Geometry check sheet. Reference: drawing and pictorial views, mm from the part's lowest x, y, z. A direction names the side the tool comes from. Give positions to 0.01 mm unless a question says otherwise; leave off trailing zeros. Order: outer loops, then holes, each group sorted by start corner. A loop starts at its lowest first (then second) coordinate and runs counter-clockwise, first axis right, second up.
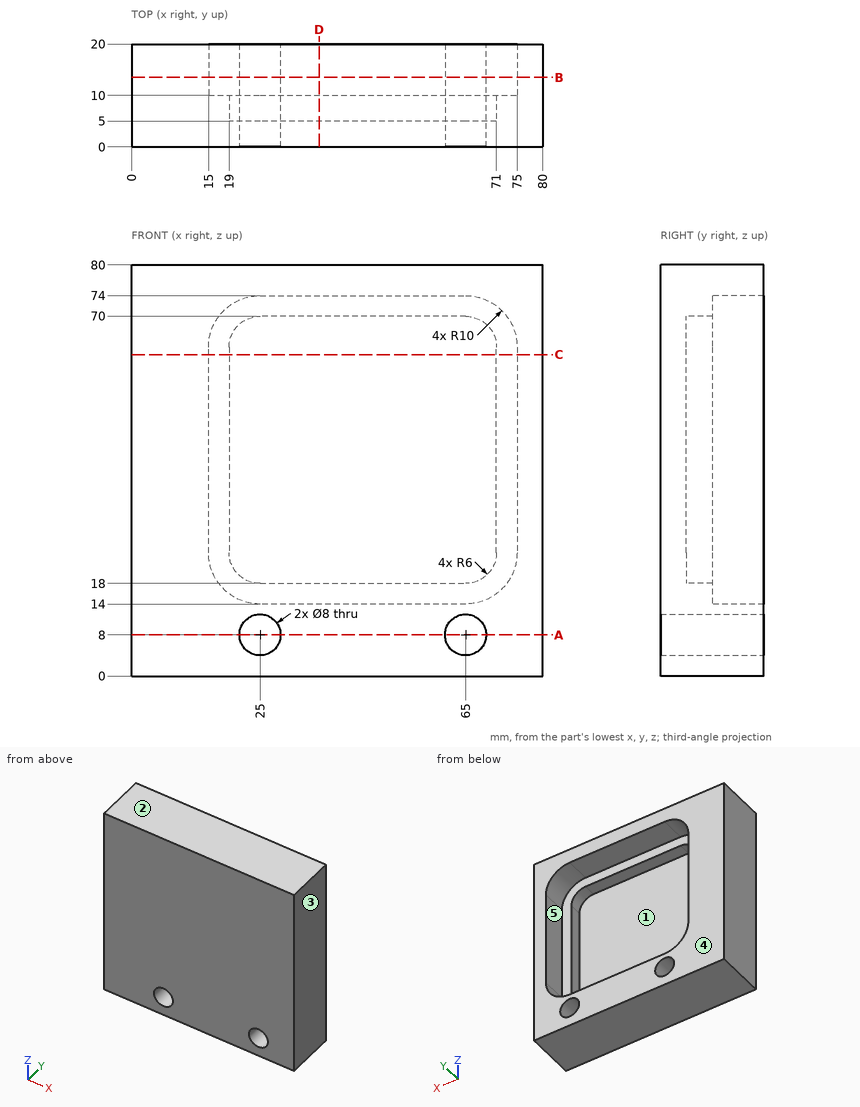
(1) Thickness scan on L1, parallel to Z at x = 25, y = 12.75; L2, parallel to Z at x = 65, y = 5.5; L3, parallel to X at y = 13.75, z = 48.5. Record the ranges inside material, lowest first.
(2) Release check for a two-part mould opening along X. For the marked faces 3, 4 and 5 record: released by +X, released by -X, zero draft, split by the parting line, or undercut.
(3) Go/stop test with a flat-tipped pin: P1, Ø6.5, axis at x = 25, z = 8, coming from the -Y side. Record where the tip stops, or that it passes through.
(4) Sectioned sample at B-B (y = 13.5). Enter the section's corners in (x, z).
(5) Sectioned sample at D-D (x = 36.5). Enter the section's corners in (y, z), plus the area to 3 significant figures.
(6) Sectioned sample at A-A (z = 8). Enter the section's corners in (x, y).
(7) Tool access check on the marked faces 1 and 2. Record the directions out of +Z, -Z, +X, -X, +Y, -Y that give a thin tool (end or side, any length) a straight path to the whole face; none if there is none.
(8) Sectioned sample at C-C (z = 62.5). Enter the section's corners in (x, y).
Values follow:
1. L1: z = 0 to 4, 12 to 14, 74 to 80
1. L2: z = 0 to 4, 12 to 18, 70 to 80
1. L3: x = 0 to 15, 75 to 80
2. face 3: released by +X
2. face 4: zero draft
2. face 5: undercut
3. P1: passes through
4. outline: (0, 0) - (80, 0) - (80, 80) - (0, 80) - close; hole (15, 24) arc R10 ccw to (25, 14) - (65, 14) arc R10 ccw to (75, 24) - (75, 64) arc R10 ccw to (65, 74) - (25, 74) arc R10 ccw to (15, 64) - close; hole circle Ø8 at (25, 8); hole circle Ø8 at (65, 8)
5. outline: (0, 0) - (20, 0) - (20, 14) - (10, 14) - (10, 18) - (5, 18) - (5, 70) - (10, 70) - (10, 74) - (20, 74) - (20, 80) - (0, 80) - close
5. area: 740 mm2
6. outline: (0, 0) - (21, 0) - (21, 20) - (0, 20) - close; (29, 0) - (61, 0) - (61, 20) - (29, 20) - close; (69, 0) - (80, 0) - (80, 20) - (69, 20) - close
7. face 1: +Y
7. face 2: +Z, +X, -X, +Y, -Y
8. outline: (0, 0) - (80, 0) - (80, 20) - (75, 20) - (75, 10) - (71, 10) - (71, 5) - (19, 5) - (19, 10) - (15, 10) - (15, 20) - (0, 20) - close
